For this review, use the dimensioned drawing (mm, ordinates from the lowest corner) and the shaded views. Coordinates: 2 decimals unless noted, no trailing zeros. Loops run counter-clockwise (first coordinate to the right, second up) from the corner with the lowest first, then second, coordinate; pieces in that order, holes last. Notation, with made-up numbers: M 52,12.25 L 100,12.25 A12 cw 100,28.25 Z; hole C 51.5,-17.75 d2. An arc over 180 degrees is marked long. Use CSV: the item, a comma, the result in double quotes. Start each with the question number.
1. Add section B-B, the plane x = 814. Write out the cut boundary in (y, z), then the cut area to 3 significant figures.
2. Add section C-C, the plane x = 991.5. Write out the cut boundary in (y, z).
3. Add section D-D, the plane z = 333.5. Write out the cut boundary in (x, y).
4. Clearance check with a flat-ended pin moving along its axis: P1, Ø17.5, axis at y = 41.5, z = 242, coming from the +X side. State where the tip first meets the part, or that it passes through.
5. Add section A-A, the plane y = 250. Write out the cut boundary in (x, z), then the cut area to 3 significant figures.
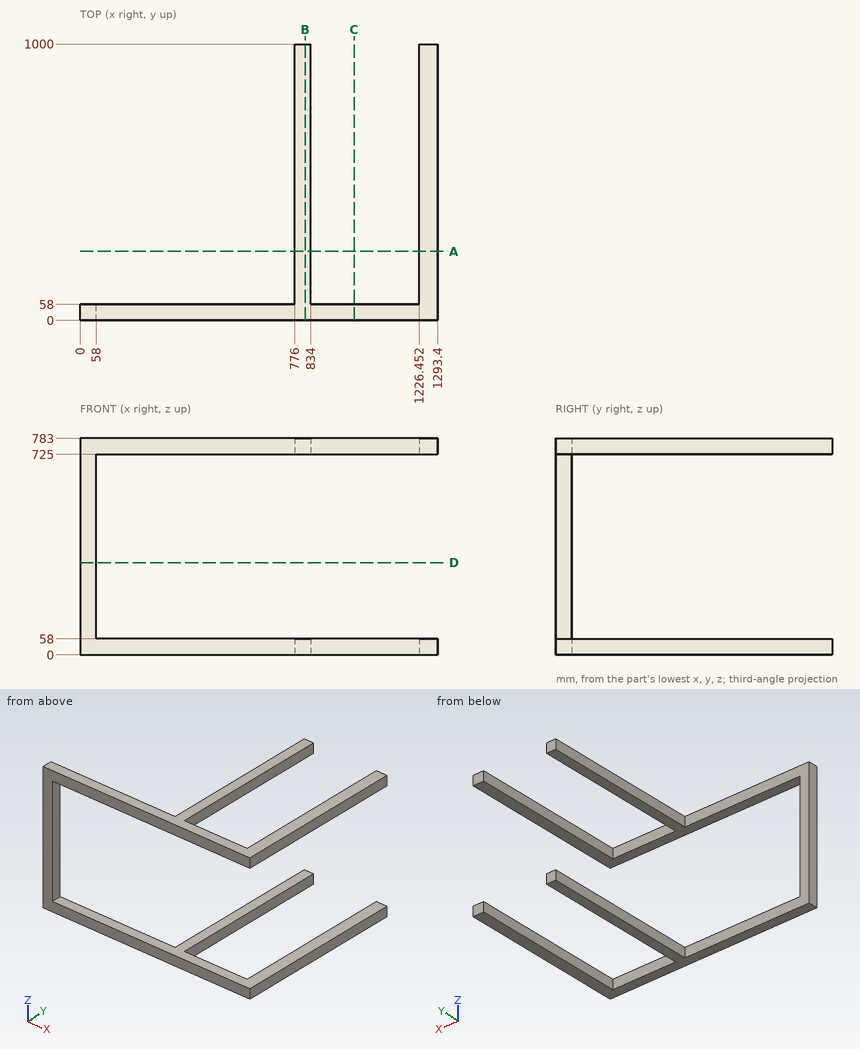
Computed:
1,outline,"M 0,0 L 1000,0 L 1000,58 L 0,58 Z; M 0,725 L 1000,725 L 1000,783 L 0,783 Z"
1,area,"116,000 mm^2"
2,outline,"M 0,0 L 58,0 L 58,58 L 0,58 Z; M 0,725 L 58,725 L 58,783 L 0,783 Z"
3,outline,"M 0,0 L 58,0 L 58,58 L 0,58 Z"
4,P1,"stops at x = 58"
5,outline,"M 776,0 L 834,0 L 834,58 L 776,58 Z; M 776,725 L 834,725 L 834,783 L 776,783 Z; M 1226.45,0 L 1293.4,0 L 1293.4,58 L 1226.45,58 Z; M 1226.45,725 L 1293.4,725 L 1293.4,783 L 1226.45,783 Z"
5,area,"14,500 mm^2"
